Can you work these out from the model? Positions are in its coordinate system, mm. A direction names the side the tool comes from. Coordinates: 2 decimals unless noted, no trailing zeros. Write each loop counter-clockwise with the first axis right and the second up, starting at its lowest first coordinate (ties: lowest second). Pieces come first, ordered by that corner, then holes. Notation, with made-up numbers: M 11.25,42.5 L 70.25,42.5 A16 ccw 70.25,49.5 Z; hole C -13.5,-4 d4. An arc over 180 degrees is marked long. Answer as a JSON object with one key per item and string values. Group by question number.
from build123d import *

# Parameters (mm, degrees)
BOSS_EXTRUDE5_DEPTH = 9.525
SKETCH5_R           = 7.9375
CUT_EXTRUDE3_DEPTH  = 4.953
SKETCH6_R           = 6.35
SKETCH6_R_2         = 2.75
CUT_EXTRUDE4_DEPTH  = 27.768093414


with BuildPart() as part:
    # Sketch2 → Boss-Extrude5 (new body)
    with BuildSketch(Plane.XY):
        with BuildLine():
            Line((-12.7, 10.16), (12.7, 10.16))
            ThreePointArc((12.7, 10.16), (22.86, 0), (12.7, -10.16))
            Line((12.7, -10.16), (-12.7, -10.16))
            ThreePointArc((-12.7, -10.16), (-22.86, 0), (-12.7, 10.16))
        make_face()
    extrude(amount=BOSS_EXTRUDE5_DEPTH)

    # Sketch5 → Cut-Extrude3 (cut)
    with BuildSketch(Plane.XY.offset(9.525)):
        Circle(SKETCH5_R)
    extrude(amount=-CUT_EXTRUDE3_DEPTH, mode=Mode.SUBTRACT)

    # Sketch6 → Cut-Extrude4 (cut, through all)
    with BuildSketch(Plane.XY.offset(9.525)):
        Circle(SKETCH6_R)
        with Locations((-12.7, 0)):
            Circle(SKETCH6_R_2)
        with Locations((12.7, 0)):
            Circle(SKETCH6_R_2)
    extrude(amount=-CUT_EXTRUDE4_DEPTH, mode=Mode.SUBTRACT)


solid = part.part
Q1. If we section it at C-C on y = -1.5: List the corners of the cut face in (x, z) for me (3 decimals).
Q2. If we section it at D-D on y = -7: List the corners of the cut face in (x, z) for me (3 decimals).
Q3. We'd pull the mould along X, two halves only. Please class faces 1 (the flat face through (0, -10.16, 5)), 2 (the cylindrical face through (-22.858, -0.223, 4.696)), 3 (the cylindrical face through (10.518, -1.673, 4.829)): pulls with the +X half, pulls with the -X half, needs draft (parallel to the pull), parting line crosses it, or undercut.
Q4. Will these pins go through, and if not, where does the flat tip stop? pin 1 (2 mm diameter, centred on x = -5.5, y = -0.5, fed in from -Z); pin 2 (2 mm diameter, centred on y = -2.5, z = 4.5, fed in from -X); pin 3 (1 mm diameter, centred on x = -16, z = 7.5, fed in from +Y).
Q5. On a 3-axis mill with a long thin cutter (end or side, diameter ignored), from which of +Z, -Z, +X, -X, +Y, -Y can I reach the whole of each face in a straight line? I mean faces 4 (the flat face through (0, 7, 4.572)), 5 (the flat face through (0, 10.16, 5)). Say none if no direction works.
Q6. Please list where these lines run through material, in increasing order: L1, parallel to Y at x = 0, z = 6.3; L2, parallel to Y at x = 12.7, z = 6.5; L3, parallel to X at y = -0.75, z = 8.5.
Q7. If we section it at B-B on z = 3.25: List the corners of the cut face in (x, y) for me.
Reply:
{
 "1": {"outline": "M -22.749,0 L -15.005,0 L -15.005,9.525 L -22.749,9.525 Z; M -10.395,0 L -6.17,0 L -6.17,4.572 L -7.794,4.572 L -7.794,9.525 L -10.395,9.525 Z; M 6.17,0 L 10.395,0 L 10.395,9.525 L 7.794,9.525 L 7.794,4.572 L 6.17,4.572 Z; M 15.005,0 L 22.749,0 L 22.749,9.525 L 15.005,9.525 Z"},
 "2": {"outline": "M -20.064,0 L 20.064,0 L 20.064,9.525 L 3.742,9.525 L 3.742,4.572 L -3.742,4.572 L -3.742,9.525 L -20.064,9.525 Z"},
 "3": {"face 1": "needs draft", "face 2": "pulls with the -X half", "face 3": "undercut"},
 "4": {"pin 1": "z = 0", "pin 2": "x = -22.75", "pin 3": "y = 9.77"},
 "5": {"face 4": "+Z", "face 5": "+Z, -Z, +X, -X, +Y"},
 "6": {"L1": "-10.16 to -7.94, 7.94 to 10.16", "L2": "-10.16 to -2.75, 2.75 to 10.16", "L3": "-22.83 to -15.35, -10.05 to -7.9, 7.9 to 10.05, 15.35 to 22.83"},
 "7": {"outline": "M -12.7,-10.16 L 12.7,-10.16 A10.16 ccw 12.7,10.16 L -12.7,10.16 A10.16 ccw Z; hole C -12.7,0 d5.5; hole C 0,0 d12.7; hole C 12.7,0 d5.5"}
}
